Check sheet for the modelled part. Datum: model origin and axes. Units: mm. A direction names the side the tool comes from. Coordinates: 2 decimals unless noted, no trailing zeros. Write each loop counter-clockwise with the first axis right and the second up, starting at its lowest first coordinate (ties: lowest second). Pieces come first, ordered by that corner, then holes. Notation, with made-up numbers: M 1.25,47.5 L 34.25,47.5 A16 ccw 34.25,56.5 Z; hole C -17,-36.75 d5. An arc over 180 degrees is marked long. Answer as CSV lines item,"result". Start each with the question number.
Q1. Depth check by flat-ended pin: pin 1 Ø5 at (x, y) = (0, 1.27) entering from +Z; pin 2 Ø1 at (y, z) = (1, 2.5) entering from -X. Enter the tip coordinate at first touch or a pass-through.
Q2. Sectioned sample at D-D, the plane y = -6.5. Record the cut outline in (x, z).
Q3. Access from +Z, -Z, +X, -X, +Y, -Y to the whole of each face (thin tool, end or side, straight path). Record for faces 4 (the flat face through (0, -3, 0)), 5 (the flat face through (4.3, 0.27, 3.5)).
Q4. Thickness scan on line 1 along Y through (x, z) = (0, 2.5); line 2 along X through (y, z) = (3.75, 3.5); line 3 along X through (y, z) = (-2, 1). Record the ranges inside material, lowest first. Write a range as from..to.
Q5. Sectioned sample at A-A, the plane x = 0. Record the cut outline in (y, z).
Q6. Sectioned sample at C-C, the plane z = 3.25. Record the cut outline in (x, y) (1 decimal), then the cut area to 3 significant figures.
Q7. Sectioned sample at B-B, the plane y = 3.5. Record the cut outline in (x, z), then the cut area to 3 significant figures.
Q8. Mould release check, pull along Y, two halves, no side actions. Record for faces 1 (the cylindrical face through (-1.72, -7.75, 3.52)), 2 (the flat face through (4.3, 2.27, 3.5)), 3 (the flat face through (0, -3, 7.144)): pulls with the +Y half, pulls with the -Y half, needs draft (parallel to the pull), parting line crosses it, or undercut.
from build123d import *

# Parameters (mm, degrees)
SKETCH1_R           = 7.9375
SKETCH1_R_2         = 4
BOSS_EXTRUDE1_DEPTH = 7.14375
CUT_EXTRUDE2_DEPTH  = 14.3056746


with BuildPart() as part:
    # Sketch1 → Boss-Extrude1 (new body)
    with BuildSketch(Plane.XY):
        Circle(SKETCH1_R)
        with Locations((0, 1.27)):
            Circle(SKETCH1_R_2, mode=Mode.SUBTRACT)
    extrude(amount=BOSS_EXTRUDE1_DEPTH)

    # Sketch8 → Cut-Extrude2 (cut, through all)
    with BuildSketch(Plane(origin=(0, 0, 0), x_dir=(-1, 0, 0), z_dir=(0, 0, -1))):
        Polygon((-4, 0.27), (-4.809500032, 0.27), (-4.809500032, 2.27), (-4, 2.27), (-3.872983346, 2.27), (-3.872983346, 0.27), align=None)
    extrude(amount=-CUT_EXTRUDE2_DEPTH, mode=Mode.SUBTRACT)


solid = part.part
Output:
1,pin 1,"passes through"
1,pin 2,"stops at x = -7.92"
2,outline,"M -4.56,0 L 4.56,0 L 4.56,7.14 L -4.56,7.14 Z"
3,face 4,"-Z, +X, -X, +Y, -Y"
3,face 5,"+Z, -Z"
4,line 1,"y = -7.94..-2.73, 5.27..7.94"
4,line 2,"x = -7..-3.14, 3.14..7"
4,line 3,"x = -7.68..-2.3, 2.3..7.68"
5,outline,"M -7.94,0 L -2.73,0 L -2.73,7.14 L -7.94,7.14 Z; M 5.27,0 L 7.94,0 L 7.94,7.14 L 5.27,7.14 Z"
6,outline,"C 0,0 d15.9; hole M 3.9,0.3 L 4.8,0.3 L 4.8,2.3 L 3.9,2.3 A4 ccw long Z"
6,area,"146 mm^2"
7,outline,"M -7.12,0 L -3.32,0 L -3.32,7.14 L -7.12,7.14 Z; M 3.32,0 L 7.12,0 L 7.12,7.14 L 3.32,7.14 Z"
7,area,"54.3 mm^2"
8,face 1,"parting line crosses it"
8,face 2,"undercut"
8,face 3,"needs draft"
